Could you check a few things on this model? Use its own coordinates, in mm. Round coordinates to 2 decimals unless told otherwise and drop trailing zeros. Loops run counter-clockwise (first coordinate to the right, second up) from the corner with the lowest first, then second, coordinate; pieces in that order, holes last. Notation, with made-up numbers: (-29, 67) -> (-21, 67) arc R8 ccw to (-21, 80) -> close; hole circle Ø5 at (-31, 1). An arc over 180 degrees is marked (long way). Write each question's results on one line, items separated by ' | '.
from build123d import *

# Parameters (mm, degrees)
SKETCH1_W                       = 50
SKETCH1_H                       = 25
SKETCH1_R                       = 1.13
BOSS_EXTRUDE1_DEPTH             = 3.175
FILLET1_R                       = 5
F_4_40_TAPPED_HOLE1_D           = 2.2606
F_4_40_TAPPED_HOLE1_ON_FACE_2_D = 2.2606


with BuildPart() as part:
    # Sketch1 → Boss-Extrude1 (new body)
    with BuildSketch(Plane(origin=(0, 0, 0), x_dir=(1, 0, 0), z_dir=(0, 1, 0))):
        with Locations((25, -12.5)):
            Rectangle(SKETCH1_W, SKETCH1_H)
        with Locations(Location((5, -5, 0), (0, 0, 270))):
            Circle(SKETCH1_R, mode=Mode.SUBTRACT)
        with Locations(Location((45, -5, 0), (0, 0, 270))):
            Circle(SKETCH1_R, mode=Mode.SUBTRACT)
        with Locations(Location((45, -20, 0), (0, 0, 270))):
            Circle(SKETCH1_R, mode=Mode.SUBTRACT)
        with Locations(Location((5, -20, 0), (0, 0, 270))):
            Circle(SKETCH1_R, mode=Mode.SUBTRACT)
    extrude(amount=BOSS_EXTRUDE1_DEPTH)

    # Fillet1
    fillet1_edges = [part.edges().sort_by_distance(p)[0] for p in [
        (0, 1.5875, 0),
        (50, 1.5875, 0),
        (50, 1.5875, 25),
        (0, 1.5875, 25),
    ]]
    fillet(fillet1_edges, radius=FILLET1_R)

    # #4-40 Tapped Hole1 (through all)
    with Locations(Plane(origin=(5, 3.175, 5), x_dir=(0, 0, 1), z_dir=(0, 1, 0))):
        with Locations((0, 0), (0, 40), (15, 40)):
            Hole(F_4_40_TAPPED_HOLE1_D / 2)

    # #4-40 Tapped Hole1 on face 2 (through all)
    with Locations(Plane(origin=(5, 0, 20), x_dir=(0, 0, 1), z_dir=(0, 1, 0))):
        with Locations((0, 0)):
            Hole(F_4_40_TAPPED_HOLE1_ON_FACE_2_D / 2)


solid = part.part
1) I want a section at A-A, the plane y = 0.85. Write out the boundary of the cut face in (x, z), plus the area to 3 significant figures.
Model answer:
outline: (0, 5) arc R5 ccw to (5, 0) -> (45, 0) arc R5 ccw to (50, 5) -> (50, 20) arc R5 ccw to (45, 25) -> (5, 25) arc R5 ccw to (0, 20) -> close; hole circle Ø2.26 at (5, 5); hole circle Ø2.26 at (5, 20); hole circle Ø2.26 at (45, 5); hole circle Ø2.26 at (45, 20) | area: 1,210 mm2
2) I'm going to push flat-ended pins straight in: pin 1 (3.5 mm diameter, centred on x = 5, z = 20, fed in from +Y) (3 decimals); pin 2 (2 mm diameter, centred on x = 5, z = 5, fed in from +Y). Where does each tip first touch, or does it pass through?
Model answer:
pin 1: stops at y = 3.175 | pin 2: passes through
3) I need wall thicknesses on line 1 (X direction, y = 2.15, z = 20); line 2 (Z direction, x = 44.5, y = 1.15); line 3 (X direction, y = 2.75, z = 22.75). Which ranges of each line are inside material? Lowest first, please.
Model answer:
line 1: x = 0 to 3.87, 6.13 to 43.87, 46.13 to 50 | line 2: z = 0 to 3.99, 6.01 to 18.99, 21.01 to 25 | line 3: x = 0.82 to 49.18
4) I want a section at B-B, the plane z = 2. Write out the boundary of the cut face in (x, y) (3 decimals), plus the area to 3 significant figures.
Model answer:
outline: (1, 0) -> (49, 0) -> (49, 3.175) -> (1, 3.175) -> close | area: 152 mm2
5) I want a section at C-C, the plane z = 22. Write out the boundary of the cut face in (x, y) (3 decimals).
Model answer:
outline: (0.417, 0) -> (49.583, 0) -> (49.583, 3.175) -> (0.417, 3.175) -> close
6) If we mould it in two halves opening along Z, with no side actions, what happens to faces 1 (the cylindrical face through (46.12, 1.57, 5.15)), 2 (the flat face through (25, 2, 25)), 3 (the flat face through (25, 2, 0))? For each: released by +Z, released by -Z, zero draft, split by the parting line, or undercut.
Model answer:
face 1: undercut | face 2: released by +Z | face 3: released by -Z
